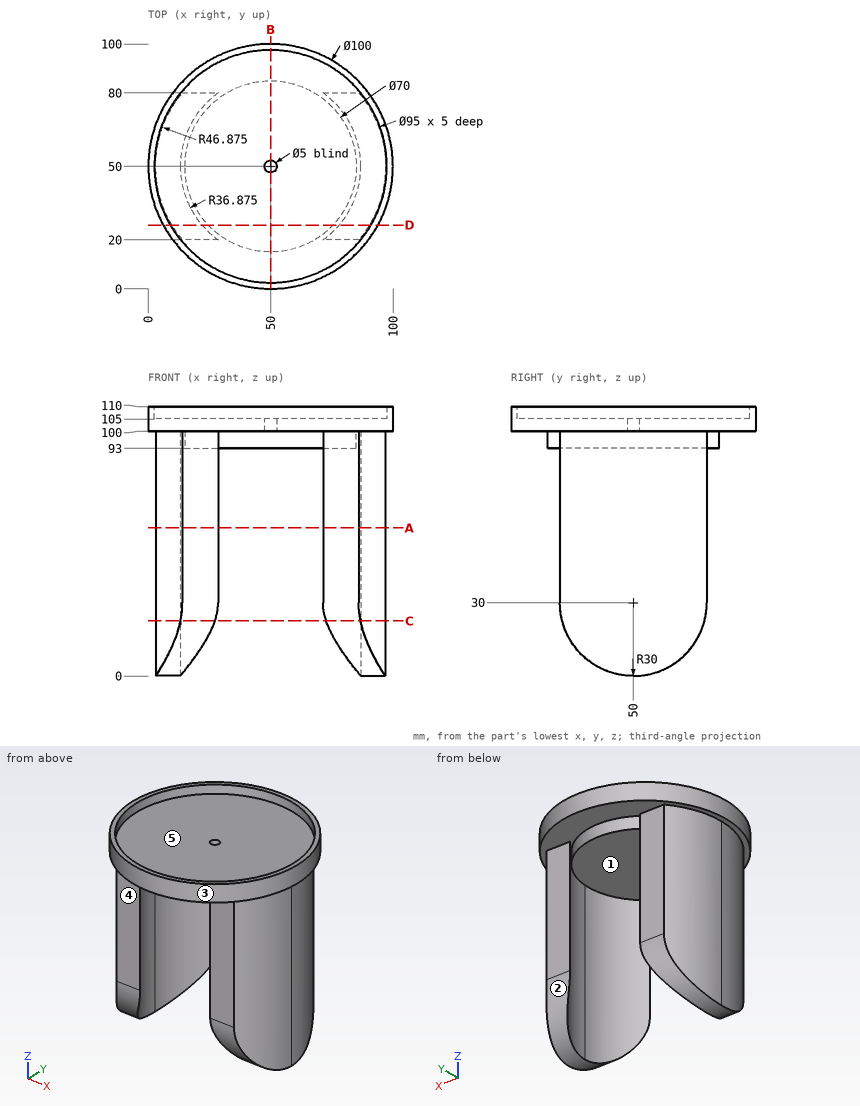
Study the drawing (mm; zero at the part's minimum x, y, z) and answer. A direction names the side the tool comes from. Give positions to 0.01 mm unless a question says otherwise; leave off trailing zeros. Write each loop counter-clockwise with the first axis right and the second up, starting at its lowest first coordinate (ties: lowest second). Pieces come first, ordered by that corner, then holes. Notation, with made-up numbers: (12, 74) -> (68, 74) arc R4 ccw to (68, 81) -> close; hole circle Ø1 at (3, 30). An arc over 180 degrees is marked (long way). Write item = value, one per line.
Q1. A tool of negligible diameter and unlimited length cuts with its end or side. For the marked faces 1 and 2, from which of +Z, -Z, +X, -X, +Y, -Y can it reach the whole face along a straight path? Write none if from no direction.
Computed values:
face_1 = -Z
face_2 = -Z, +X, -X
Q2. Section B-B on x = 50 is taken. Determine the outline of the cut face in (y, z).
Computed values:
outline = (0, 100) -> (15, 100) -> (15, 93) -> (85, 93) -> (85, 100) -> (100, 100) -> (100, 110) -> (97.5, 110) -> (97.5, 105) -> (52.5, 105) -> (52.5, 100) -> (47.5, 100) -> (47.5, 105) -> (2.5, 105) -> (2.5, 110) -> (0, 110) -> close
Q3. Consider line 1 along Y through (x, z) = (50, 107.1); line 2 along X through (y, z) = (61, 16); line 3 along Z through (x, y) = (40, 91). Determine where each line is inside the solid, lowest interval first.
Computed values:
line_1 = 0 to 2.5, 97.5 to 100
line_2 = 4.43 to 14.8, 85.2 to 95.57
line_3 = 100 to 105
Q4. Flat-ended cylindrical pins translate along their axes: pin 1 Ø16 at (x, z) = (18.5, 49) entering from -Y; pin 2 Ø6 at (x, y) = (44, 80) entering from +Z; pin 3 Ø4.5 at (x, z) = (20, 78) entering from +Y. Find the tip coordinate at first contact, or state that the pin passes through.
Computed values:
pin_1 = 20
pin_2 = 105
pin_3 = 80
Q5. For a pull along X with two mould halves and no side action, classify the marked faces 3, 4 and 5 as pulls with the +X half, pulls with the -X half, needs draft (parallel to the pull), parting line crosses it, or undercut.
Computed values:
face_3 = parting line crosses it
face_4 = needs draft
face_5 = undercut
Q6. Section A-A on z = 60.5 is taken. Determine the outline of the cut face in (x, y) (3 decimals), and give its area (3 significant figures).
Computed values:
outline = (13.982, 20) -> (28.558, 20) arc R36.875 cw to (28.558, 80) -> (13.982, 80) arc R46.875 ccw to start; (71.442, 20) -> (86.018, 20) arc R46.875 ccw to (86.018, 80) -> (71.442, 80) arc R36.875 cw to start
area = 1,340 mm^2
Q7. Section D-D on y = 26 is taken. Determine the outline of the cut face in (x, z), and give its area (3 significant figures).
Computed values:
outline = (6.14, 100) -> (9.74, 100) -> (9.74, 12) -> (22, 12) -> (22, 100) -> (24.52, 100) -> (24.52, 93) -> (75.48, 93) -> (75.48, 100) -> (78, 100) -> (78, 12) -> (90.26, 12) -> (90.26, 100) -> (93.86, 100) -> (93.86, 110) -> (90.99, 110) -> (90.99, 105) -> (9.01, 105) -> (9.01, 110) -> (6.14, 110) -> close
area = 2,980 mm^2
Q8. Section C-C on z = 22.5 is taken. Determine the outline of the cut face in (x, y) (3 decimals), and give its area (3 significant figures).
Computed values:
outline = (13.21, 20.953) -> (27.284, 20.953) arc R36.875 cw to (27.284, 79.047) -> (13.21, 79.047) arc R46.875 ccw to start; (72.716, 20.953) -> (86.79, 20.953) arc R46.875 ccw to (86.79, 79.047) -> (72.716, 79.047) arc R36.875 cw to start
area = 1,290 mm^2
